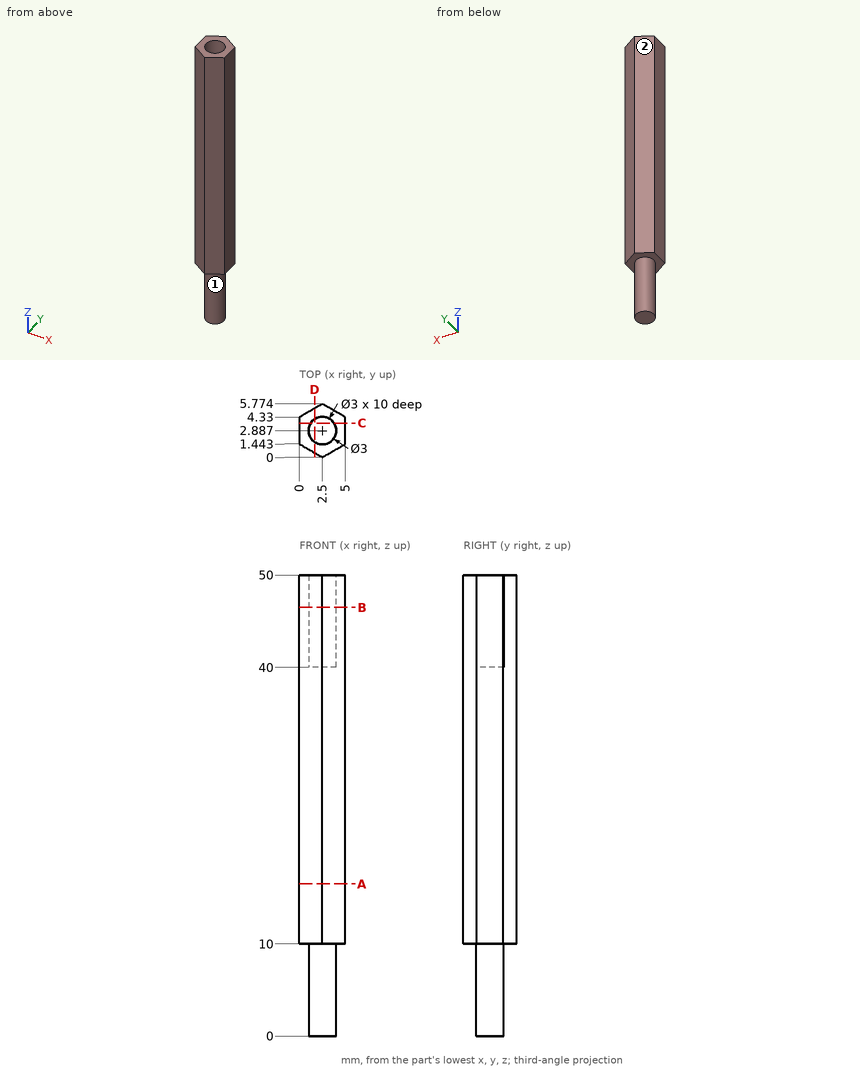
Geometry check sheet. Reference: drawing and pictorial views, mm from the part's lowest x, y, z. A direction names the side the tool comes from. Coordinates: 2 decimals unless noted, no trailing zeros. Order: outer loops, then holes, each group sorted by start corner. A loop starts at its lowest first (then second) coordinate and runs counter-clockwise, first axis right, second up.
Item 1: Tool access check on the marked faces 1 and 2. Record the directions out of +Z, -Z, +X, -X, +Y, -Y that give a thin tool (end or side, any length) a straight path to the whole face; none if there is none.
Item 2: Scan lines: line 1 along Y through (x, z) = (2.5, 42.75) (1 decimal); line 2 along Z through (x, y) = (2.45, 0.85); line 3 along Z through (x, y) = (3.4, 2.4). Record each from-to range of solid material in increasing order.
Item 3: Section check D-D (x = 1.65). Enter the section's corners in (y, z), plus the area to 3 significant figures.
Item 4: Section check A-A (z = 16.5). Enter the section's corners in (x, y).
Item 5: Section check C-C (y = 3.7). Enter the section's corners in (x, z), plus the area to 3 significant figures.
Item 6: Section check B-B (z = 46.5). Enter the section's corners in (x, y), plus the area to 3 significant figures.
Item 7: Depth check by flat-ended pin: pin 1 (2 mm diameter, centred on x = 4.5, y = 1, fed in from -Z); pin 2 (2 mm diameter, centred on y = 3, z = 18, fed in from -X); pin 3 (1.8 mm diameter, centred on x = 2.5, y = 2.89, fed in from +Z); pin 4 (2 mm diameter, centred on x = 1, z = 44.5, fed in from -Y). Enter the tip coordinate at first touch or a pass-through.
Check sheet entries:
1. face 1: -Z
1. face 2: +Z, -Z, -X, +Y
2. line 1: y = 0 to 1.4, 4.4 to 5.8
2. line 2: z = 10 to 50
2. line 3: z = 0 to 40
3. outline: (0.49, 10) - (1.65, 10) - (1.65, 0) - (4.12, 0) - (4.12, 10) - (5.28, 10) - (5.28, 50) - (4.12, 50) - (4.12, 40) - (1.65, 40) - (1.65, 50) - (0.49, 50) - close
3. area: 192 mm2
4. outline: (0, 1.44) - (2.5, 0) - (5, 1.44) - (5, 4.33) - (2.5, 5.77) - (0, 4.33) - close
5. outline: (0, 10) - (1.24, 10) - (1.24, 0) - (3.76, 0) - (3.76, 10) - (5, 10) - (5, 50) - (3.76, 50) - (3.76, 40) - (1.24, 40) - (1.24, 50) - (0, 50) - close
5. area: 200 mm2
6. outline: (0, 1.44) - (2.5, 0) - (5, 1.44) - (5, 4.33) - (2.5, 5.77) - (0, 4.33) - close; hole circle Ø3 at (2.5, 2.89)
6. area: 14.6 mm2
7. pin 1: stops at z = 10
7. pin 2: stops at x = 0
7. pin 3: stops at z = 40
7. pin 4: stops at y = 0.29
